Geometry: final body of the model. Coordinates: model frame, mm. Face numbers are marked on the shaded views. A direction names the side the tool comes from. Coordinates: 2 decimals unless noted, no trailing zeros. Loops run counter-clockwise (first coordinate to the right, second up) from the corner with the lowest first, then second, coordinate; pieces in that order, holes last. Notation, with made-up numbers: (80, 53.5) - (101, 53.5) arc R26 ccw to (101, 81.5) - close; hole circle Ø10 at (-18.75, 82.5). An arc over 180 degrees is marked (long way). Return JSON: item names as keys, results as strings.
from build123d import *

# Parameters (mm, degrees)
SKETCH1_R           = 11
BOSS_EXTRUDE1_DEPTH = 5.925
SKETCH2_R           = 25
BOSS_EXTRUDE2_DEPTH = 3.175
SKETCH3_R           = 2.54
CUT_EXTRUDE1_DEPTH  = 36.848369907


with BuildPart() as part:
    # Sketch1 → Boss-Extrude1 (new body)
    with BuildSketch(Plane(origin=(0, 0, 0), x_dir=(0, 0, -1), z_dir=(1, 0, 0))):
        Circle(SKETCH1_R)
        with BuildLine():
            Line((-5.25, 3.391164992), (-5.25, -3.391164992))
            ThreePointArc((-5.25, -3.391164992), (0, -6.25), (5.25, -3.391164992))
            Line((5.25, -3.391164992), (5.25, 3.391164992))
            ThreePointArc((5.25, 3.391164992), (0, 6.25), (-5.25, 3.391164992))
        make_face(mode=Mode.SUBTRACT)
    extrude(amount=BOSS_EXTRUDE1_DEPTH)

    # Sketch2 → Boss-Extrude2 (add)
    with BuildSketch(Plane(origin=(5.925, 0, 0), x_dir=(0, 0, -1), z_dir=(1, 0, 0))):
        Circle(SKETCH2_R)
        with BuildLine():
            Line((-5.25, 3.391164992), (-5.25, -3.391164992))
            ThreePointArc((-5.25, -3.391164992), (0, -6.25), (5.25, -3.391164992))
            Line((5.25, -3.391164992), (5.25, 3.391164992))
            ThreePointArc((5.25, 3.391164992), (0, 6.25), (-5.25, 3.391164992))
        make_face(mode=Mode.SUBTRACT)
    extrude(amount=BOSS_EXTRUDE2_DEPTH)

    # Sketch3 → Cut-Extrude1 (cut, through all)
    with BuildSketch(Plane.ZY.offset(-5.925)):
        with Locations((0, 18)):
            Circle(SKETCH3_R)
        with Locations((17.119017293, 5.562305899)):
            Circle(SKETCH3_R)
        with Locations((10.580134541, -14.562305899)):
            Circle(SKETCH3_R)
        with Locations((-10.580134541, -14.562305899)):
            Circle(SKETCH3_R)
        with Locations((-17.119017293, 5.562305899)):
            Circle(SKETCH3_R)
    extrude(amount=-CUT_EXTRUDE1_DEPTH, mode=Mode.SUBTRACT)


solid = part.part
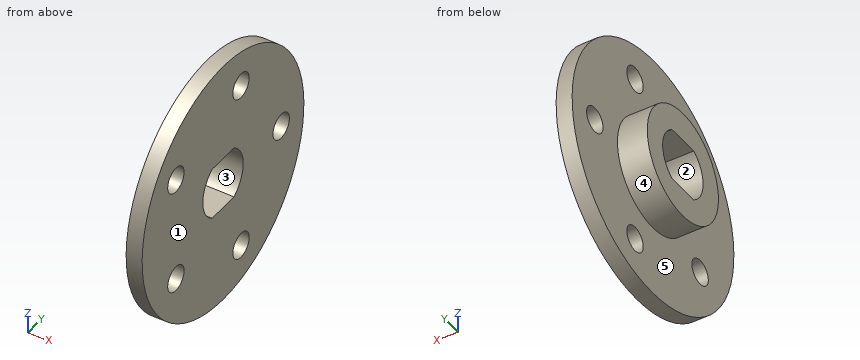
Item 1: Mould query, pull axis Y, two halves, no side actions, for the marked faces 3, 4 and 5. Classes: +Y half, -Y half, draft (parallel to the pull), parting line (faces both ways), or undercut.
Worked out:
{"face 3": "undercut", "face 4": "parting line", "face 5": "draft"}
Item 2: Section query B-B, the plane z = 0. Return loops of the section in (x, y) (3 decimals), and give its area (3 significant figures).
Worked out:
{"outline": "(0, -11) - (5.925, -11) - (5.925, -25) - (9.1, -25) - (9.1, -6.25) - (0, -6.25) - close; (0, 6.25) - (9.1, 6.25) - (9.1, 15.46) - (5.925, 15.46) - (5.925, 11) - (0, 11) - close; (5.925, 20.54) - (9.1, 20.54) - (9.1, 25) - (5.925, 25) - close", "area": "159 mm^2"}
Item 3: First-contact query: pin 1 Ø2 at (x, y) = (2.5, -13) entering from +Z; pin 2 Ø6 at (y, z) = (-14.56, 10.58) entering from -X (3 decimals); pin 3 Ø1.5 at (x, z) = (6, 9.5) entering from -Y; pin 4 Ø3 at (x, y) = (5, 9.5) entering from +Z. Flat tips, straight axial feed; report the tip coordinate or a pass-through.
Worked out:
{"pin 1": "through", "pin 2": "x = 5.925", "pin 3": "y = -23.42", "pin 4": "z = 23.58"}
Item 4: Section query C-C, the plane z = -10. Return loops of the section in (x, y) (3 decimals).
Worked out:
{"outline": "(0, -4.583) - (5.925, -4.583) - (5.925, -12.089) - (9.1, -12.089) - (9.1, 22.913) - (5.925, 22.913) - (5.925, 4.583) - (0, 4.583) - close; (5.925, -22.913) - (9.1, -22.913) - (9.1, -17.035) - (5.925, -17.035) - close"}
Item 5: Section query A-A, the plane y = 0. Return loops of the section in (x, z) (3 decimals).
Worked out:
{"outline": "(0, -11) - (5.925, -11) - (5.925, -25) - (9.1, -25) - (9.1, -5.25) - (0, -5.25) - close; (0, 5.25) - (9.1, 5.25) - (9.1, 25) - (5.925, 25) - (5.925, 11) - (0, 11) - close"}
Item 6: Section query D-D, the plane x = 3.5. Return loops of the section in (y, z).
Worked out:
{"outline": "circle Ø22 at (0, 0); hole (-3.39, -5.25) - (3.39, -5.25) arc R6.25 ccw to (3.39, 5.25) - (-3.39, 5.25) arc R6.25 ccw to start"}
Item 7: Ray query, probe 1 along Y at (x, z) = (7.7, 0); probe 2 along Z at (x, y) = (7.75, 5); probe 3 along Z at (x, y) = (8, -15.5). Return the intervals inside material, ascending. Write a range as from..to.
Worked out:
{"probe 1": "-25..-6.25, 6.25..15.46, 20.54..25", "probe 2": "-24.49..-19.6, -14.64..-3.75, 3.75..14.64, 19.6..24.49", "probe 3": "-19.62..-12.94, -8.22..8.22, 12.94..19.62"}
Item 8: Reachability of the marked faces 1 and 2 from +Z, -Z, +X, -X, +Y, -Y: full face, straight path, thin tool, end or side. Return the list, or none.
Worked out:
{"face 1": "+Z, -Z, +X, +Y, -Y", "face 2": "+X, -X"}
